Source: CAD feature listing. Evaluate the final solid. Frame: model axes, mm. Face numbers are marked on the shaded views. Round coordinates to 2 decimals unless told otherwise and drop trailing zeros. Order: outer loops, then holes, each group sorted by start corner. A loop starts at its lowest first (then second) coordinate and runs counter-clockwise, first axis right, second up. Notation, with made-up numbers: M 4.25,83.5 L 20.25,83.5 A16 ccw 20.25,111.5 Z; hole C 14,37 d11. An arc over 180 degrees is marked long. Use one line per item in the form item = value. Start each with the question number.
Q1. Section C-C (x = 25.4). Return the cut outline in (y, z) (1 decimal), plus the area to 3 significant figures.
Q2. Section A-A (y = -13). Return the cut outline in (x, z) (3 decimals), plus the area to 3 significant figures.
Q3. Pull-direction query (X, two-part tool) for the marked faces 1 and 2; classes: pulls with the +X half, pulls with the -X half, needs draft (parallel to the pull), parting line crosses it, or undercut.
Q4. Contact query for flat-ended pins moving along their axis: pin 1 (5 mm diameter, centred on x = 25.4, z = 10.16, fed in from +Y); pin 2 (2 mm diameter, centred on x = 30, y = 14, fed in from -Z); pin 3 (6 mm diameter, centred on x = 28.5, y = 20.5, fed in from +Z). Output: stop coordinate, or through.
Q5. Section D-D (z = 5.5). Return the cut outline in (x, y), plus the area to 3 significant figures.
Q6. Material intervals for probe 1 along X at (y, z) = (19, 10.16) (3 decimals); probe 2 along Y at (x, z) = (-38, 18); probe 3 along X at (y, z) = (28, 12.5), sorted ascending.
from build123d import *

# Parameters (mm, degrees)
BOSS_EXTRUDE1_DEPTH = 20.32
SKETCH2_R           = 6.35
SKETCH2_R_2         = 3.175
BOSS_EXTRUDE2_DEPTH = 50.8


with BuildPart() as part:
    # Sketch1 → Boss-Extrude1 (new body)
    with BuildSketch(Plane.XY):
        Polygon((-44.173002637, -17.9705), (44.173002637, -17.9705), (42.424083396, -21.7805), (-42.424083396, -21.7805), align=None)
    extrude(amount=BOSS_EXTRUDE1_DEPTH)

    # Sketch2 → Boss-Extrude2 (add)
    # profile 1 of 2: a face of its own
    with BuildSketch(Plane(origin=(0, -17.9705, 0), x_dir=(1, 0, 0), z_dir=(0, 1, 0))):
        with Locations(Location((-25.4, -10.16, 0), (0, 0, 90))):
            Circle(SKETCH2_R)
        with Locations(Location((-25.4, -10.16, 0), (0, 0, 270))):
            Circle(SKETCH2_R_2, mode=Mode.SUBTRACT)
    # profile 2 of 2: a face of its own
    with BuildSketch(Plane(origin=(0, -17.9705, 0), x_dir=(1, 0, 0), z_dir=(0, 1, 0))):
        with Locations(Location((25.4, -10.16, 0), (0, 0, 90))):
            Circle(SKETCH2_R)
        with Locations(Location((25.4, -10.16, 0), (0, 0, 270))):
            Circle(SKETCH2_R_2, mode=Mode.SUBTRACT)
    extrude(amount=BOSS_EXTRUDE2_DEPTH)


solid = part.part
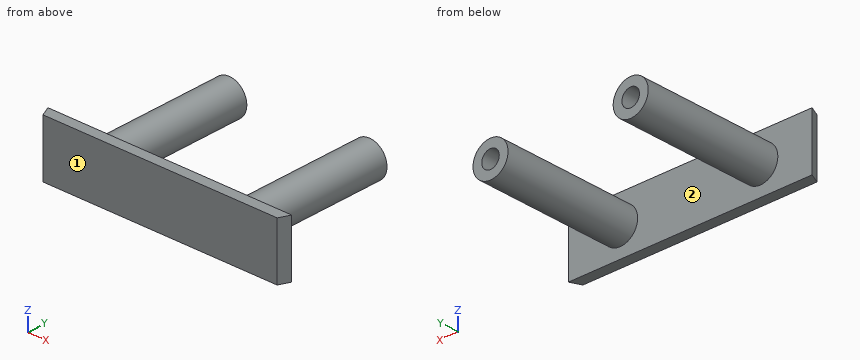
Results list:
q1.outline = M -21.8,0 L -18,0 L -18,3.8 L 32.8,3.8 L 32.8,7 L -18,7 L -18,13.3 L 32.8,13.3 L 32.8,16.5 L -18,16.5 L -18,20.3 L -21.8,20.3 Z
q1.area = 400 mm2
q2.outline = C -25.4,10.16 d12.7; C 25.4,10.16 d12.7; hole C -25.4,10.16 d6.35; hole C 25.4,10.16 d6.35
q2.area = 190 mm2
q3.face_1 = needs draft
q3.face_2 = undercut
q4.pin_1 = -17.97
q4.pin_2 = 4.93
q4.pin_3 = 16.51
q5.outline = M -44.17,-17.97 L -42.42,-21.78 L 42.42,-21.78 L 44.17,-17.97 L 29.71,-17.97 L 29.71,32.83 L 21.09,32.83 L 21.09,-17.97 L -21.09,-17.97 L -21.09,32.83 L -29.71,32.83 L -29.71,-17.97 Z
q5.area = 1,210 mm2
q6.probe_1 = -31.75 to -28.575, -22.225 to -19.05, 19.05 to 22.225, 28.575 to 31.75
q6.probe_2 = -21.78 to -17.97
q6.probe_3 = -31.3 to -27.55, -23.25 to -19.5, 19.5 to 23.25, 27.55 to 31.3
